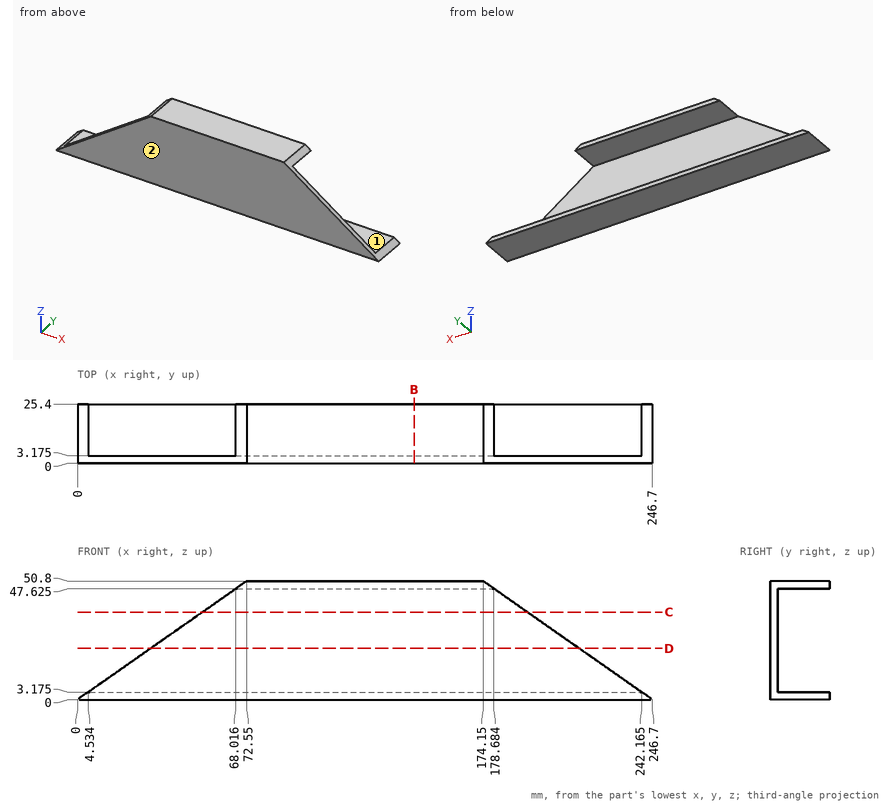
Print and shaded views of the part. All mm, measured from the part's lowest x, y and z. A direction names the side the tool comes from. Coordinates: 2 decimals unless noted, no trailing zeros. Loops run counter-clockwise (first coordinate to the right, second up) from the corner with the lowest first, then second, coordinate; pieces in that order, holes last. Notation, with made-up numbers: (-13, 66) - (17, 66) arc R9 ccw to (17, 82) - close; hole circle Ø7 at (12, -22.5). An arc over 180 degrees is marked (long way). Write item = value, one per line. Start each with the question number.
Item 1: 3-axis set-ups, long thin cutter, end or side, ignore diameter. For the marked faces 1 and 2: which of +Z, -Z, +X, -X, +Y, -Y reach the whole face in a straight line?
Item 2: Saw through at C-C, the plane z = 37.5. List the corners of the cut face in (x, y) (1 decimal).
Item 3: Wall check: probe 1 along Z at (x, y) = (166, 10.5) (1 decimal); probe 2 along Y at (x, z) = (60.5, 28.5) (1 decimal). Give the ranges that are in metal, low to high. Write a range as [from, to].
Item 4: Saw through at D-D, the plane z = 22. List the corners of the cut face in (x, y) (1 decimal).
Item 5: Drop flat-ended pins along their axis: pin 1 Ø5 at (x, z) = (161, 41.5) entering from +Y (3 decimals); pin 2 Ø8 at (x, y) = (28.5, 20) entering from +Z (3 decimals). Give the stop position or say it passes through.
Item 6: Saw through at B-B, the plane x = 144.5. List the corners of the cut face in (y, z) (1 decimal).
Answers:
q1.face_1 = +X, -X, +Y
q1.face_2 = +Z, -Z, +X, -X, -Y
q2.outline = (53.6, 0) - (193.1, 0) - (193.1, 3.2) - (53.6, 3.2) - close
q3.probe_1 = [0, 3.2], [47.6, 50.8]
q3.probe_2 = [0, 3.2]
q4.outline = (31.4, 0) - (215.3, 0) - (215.3, 3.2) - (31.4, 3.2) - close
q5.pin_1 = 3.175
q5.pin_2 = 3.175
q6.outline = (0, 0) - (25.4, 0) - (25.4, 3.2) - (3.2, 3.2) - (3.2, 47.6) - (25.4, 47.6) - (25.4, 50.8) - (0, 50.8) - close
